Geometry: see drawing. Coordinates: mm, zero at the bounding-box minimum. Coordinates: 2 decimals unless noted, no trailing zeros. Order: outer loops, then holes, each group sorted by start corner. A loop starts at its lowest first (then second) coordinate and runs counter-clockwise, first axis right, second up.
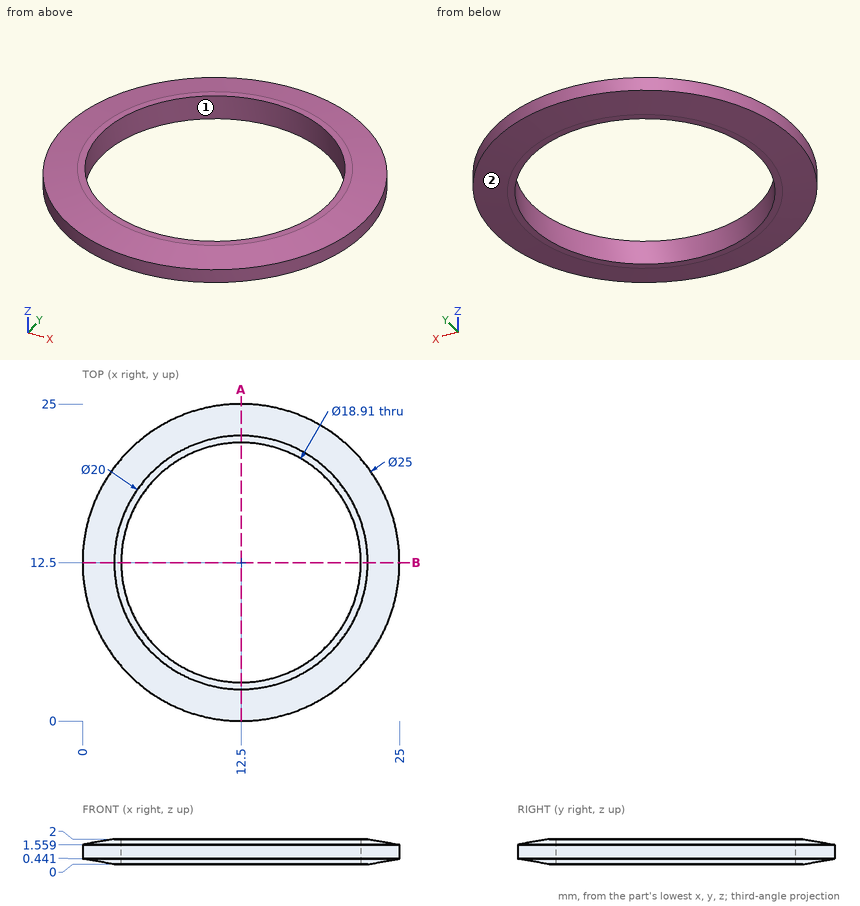
Item 1: Pin query (flat end, axial travel): pin 1 Ø6 at (x, y) = (5.5, 11) entering from -Z. Return the tip coordinate at first contact, or that it passes through.
Response values:
pin 1: stops at z = 0
Item 2: Draft query along Y for the marked faces 1 and 2. Return one class per face: pulls with the +Y half, pulls with the -Y half, needs draft (parallel to the pull), parting line crosses it, or undercut.
Response values:
face 1: undercut
face 2: parting line crosses it
Item 3: Ray query, probe 1 along Y at (x, z) = (12.5, 0.9) (3 decimals); probe 2 along X at (y, z) = (18, 0.9) (1 decimal); probe 3 along X at (y, z) = (16.5, 0.55). Return the intervals inside material, ascending.
Response values:
probe 1: y = 0 to 3.045, 21.955 to 25
probe 2: x = 1.3 to 4.8, 20.2 to 23.7
probe 3: x = 0.66 to 3.93, 21.07 to 24.34
Item 4: Cut plane A-A on x = 12.5. Return loops of the section in (y, z) (1 decimal).
Response values:
outline: (0, 0.4) - (2.5, 0) - (3, 0) - (3, 2) - (2.5, 2) - (0, 1.6) - close; (22, 0) - (22.5, 0) - (25, 0.4) - (25, 1.6) - (22.5, 2) - (22, 2) - close
